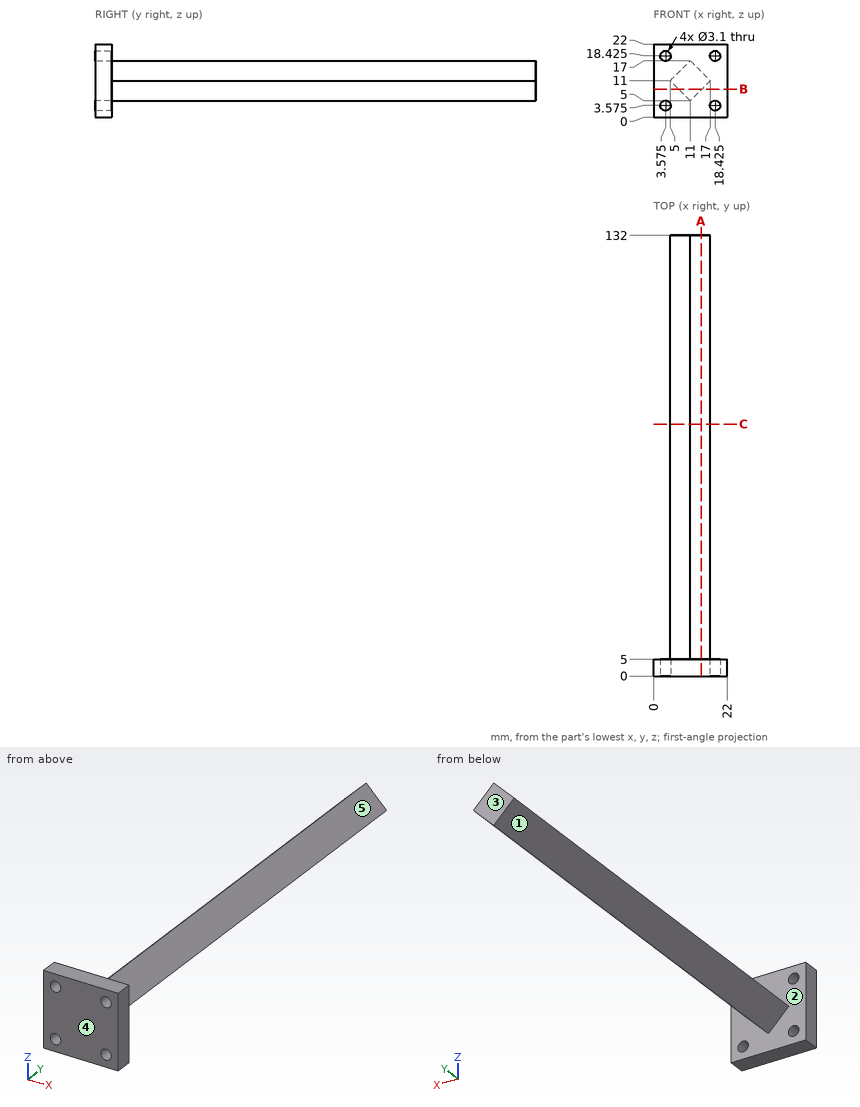
Geometry: see drawing. Coordinates: mm, zero at the bounding-box minimum. A direction names the side the tool comes from. Coordinates: 2 decimals unless noted, no trailing zeros. Order: outer loops, then holes, each group sorted by start corner. A loop starts at its lowest first (then second) coordinate and runs counter-clockwise, first axis right, second up. Notation, with made-up numbers: (-26, -15.75) - (-1, -15.75) arc R12 ccw to (-1, -2.75) - close; hole circle Ø9 at (78.5, 19.25). An arc over 180 degrees is marked (long way). Write each question's results on one line, items separated by ' | '.
1) Line query: line 1 (Y direction, x = 8, z = 20.5); line 2 (Z direction, x = 16, y = 126.5); line 3 (Z direction, x = 11.5, y = 123). Output: solid intervals per line, ascending. Write a range as from..to.
Results list:
line 1: 0..5 | line 2: 10..12 | line 3: 5.5..16.5
2) Pin query (flat end, axial travel): pin 1 (5 mm diameter, centred on x = 18.42, z = 3.58, fed in from +Y); pin 2 (3 mm diameter, centred on y = 98.5, z = 11, fed in from +X); pin 3 (4 mm diameter, centred on y = 43.5, z = 18.5, fed in from +X). Return the tip coordinate at first contact, or that it passes through.
Results list:
pin 1: y = 5 | pin 2: x = 17 | pin 3: x = 11.5
3) Section C-C, the plane y = 75.5. Return loops of the section in (x, z), plus the area to 3 significant figures.
Results list:
outline: (5, 11) - (11, 5) - (17, 11) - (11, 17) - close | area: 72.0 mm^2
4) Section A-A, the plane x = 14.25. Return loops of the section in (y, z).
Results list:
outline: (0, 0) - (5, 0) - (5, 8.25) - (132, 8.25) - (132, 13.75) - (5, 13.75) - (5, 22) - (0, 22) - close
5) Section B-B, the plane z = 8.5. Return loops of the section in (x, y).
Results list:
outline: (0, 0) - (22, 0) - (22, 5) - (14.5, 5) - (14.5, 132) - (7.5, 132) - (7.5, 5) - (0, 5) - close
6) Set-up query: the marked faces 1, 2, 3, 4 and 5. Return all of +Z, -Z, +X, -X, +Y, -Y with unobstructed straight access to the full face (end or side cutting, diameter ignored); none if empty.
Results list:
face 1: -Z, -X, +Y | face 2: +Y | face 3: +Z, -Z, +X, -X, +Y | face 4: +Z, -Z, +X, -X, -Y | face 5: +Z, +X, +Y
